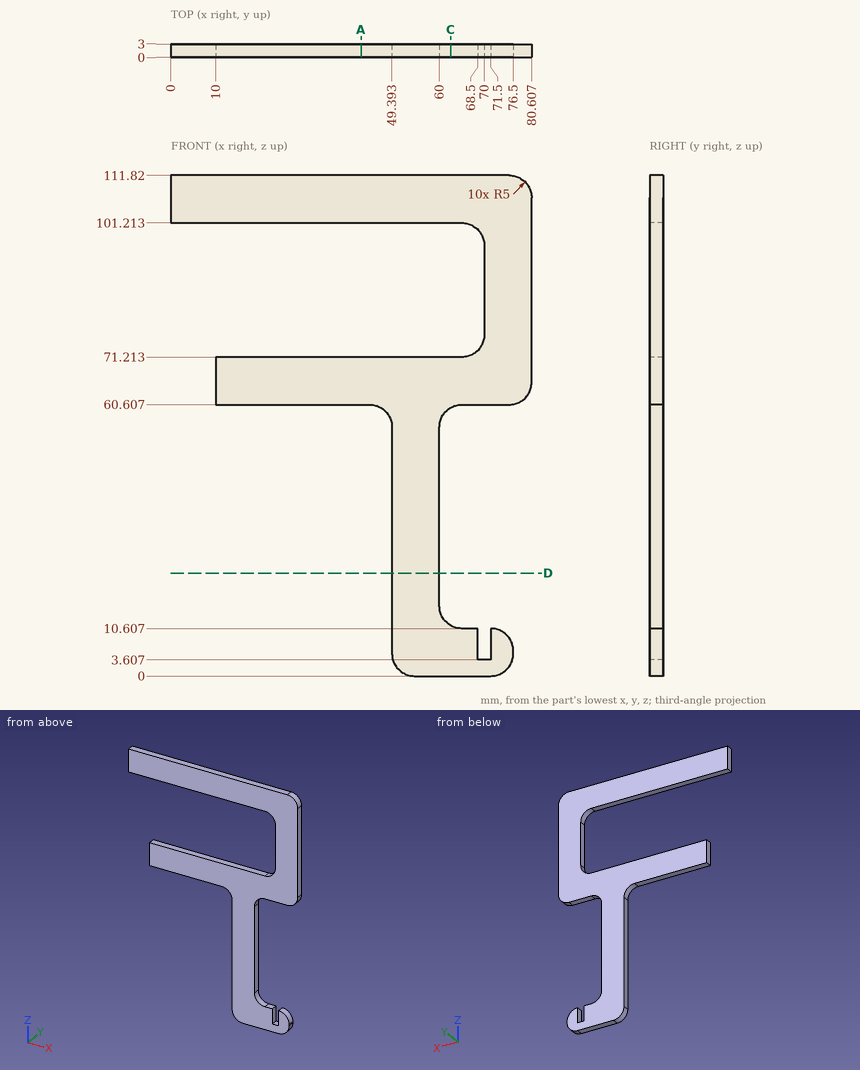
The drawing under review shows one solid part. Ordinate dimensions are in mm from its lowest x, y, z. Round coordinates to 2 decimals unless told otherwise and drop trailing zeros. Write each loop counter-clockwise with the first axis right and the second up, starting at its lowest first coordinate (ties: lowest second). Pieces come first, ordered by that corner, then holes. Notation, with made-up numbers: (2.5, 32.5) - (18.5, 32.5) arc R11 ccw to (18.5, 47.5) - close; hole circle Ø4 at (85.25, 34). An arc over 180 degrees is marked (long way). Write each question's results on one line, items separated by ' | '.
Item 1: Take a section at A-A on x = 42.5. State the section outline as (y, z) points.
Calculated:
outline: (0, 60.61) - (3, 60.61) - (3, 71.21) - (0, 71.21) - close; (0, 101.21) - (3, 101.21) - (3, 111.82) - (0, 111.82) - close
Item 2: Take a section at D-D on z = 23. State the section outline as (x, y) points, then the cut area to 3 significant figures.
Calculated:
outline: (49.39, 0) - (60, 0) - (60, 3) - (49.39, 3) - close | area: 31.8 mm^2
Item 3: For pin 1 (1.5 mm diameter, centred on y = 2, z = 59, fed in from +X); pin 2 (0.9 mm diameter, centred on y = 2, z = 39, fed in from -X); pin 3 (0.7 mm diameter, centred on y = 2, z = 5.5, fed in from +X), all flat-tipped, find the tip position at first contact; note any pin that passes through.
Calculated:
pin 1: stops at x = 62.2 | pin 2: stops at x = 49.39 | pin 3: stops at x = 76.5
Item 4: Take a section at C-C on x = 62.5. State the section outline as (y, z) points.
Calculated:
outline: (0, 0) - (3, 0) - (3, 11.28) - (0, 11.28) - close; (0, 59.94) - (3, 59.94) - (3, 71.21) - (0, 71.21) - close; (0, 101.21) - (3, 101.21) - (3, 111.82) - (0, 111.82) - close
Item 5: To check wall thickness, follow line 1 along Z through (x, y) = (38.5, 2.4); line 2 along Z through (x, y) = (54.5, 2); line 3 along X through (y, z) = (0.7, 48). State the ranges of each line that lie inside material, in increasing order. Write a range as from..to.
Calculated:
line 1: z = 60.61..71.21, 101.21..111.82 | line 2: z = 0..71.21, 101.21..111.82 | line 3: x = 49.39..60
